from build123d import *

# Parameters (mm, degrees)
F1_DEPTH = 16
F2_R     = 5
F3_DEPTH = 31.200998


with BuildPart() as f1:
    # F0 (on Top) → F1 (new body)
    with BuildSketch(Plane.XY):
        with BuildLine():
            Line((-49.38504, 20.824596), (-48.185041, 20.824596))
            Line((-48.185041, 20.824596), (-48.185041, 36.824596))
            ThreePointArc((-48.185041, 36.824596), (-46.427682, 41.067237), (-42.185041, 42.824596))
            Line((-42.185041, 42.824596), (-18.185041, 42.824596))
            Line((-18.185041, 42.824596), (-18.185041, 44.024594))
            Line((-18.185041, 44.024594), (-42.185041, 44.024594))
            ThreePointArc((-42.185041, 44.024594), (-47.276209, 41.915763), (-49.38504, 36.824596))
            Line((-49.38504, 36.824596), (-49.38504, 20.824596))
        make_face()
    extrude(amount=F1_DEPTH)

    # F2 (on face) → F3 (cut, through all)
    with BuildSketch(Plane(origin=(-49.38504, 0, 0), x_dir=(0, -1, 0), z_dir=(-1, 0, 0))):
        with Locations((-28.824596, 8)):
            Circle(F2_R)
    extrude(amount=-F3_DEPTH, mode=Mode.SUBTRACT)


solid = f1.part
Verification items for the finished model (mm, model axes). A direction names the side the tool comes from. Coordinates: 2 decimals unless noted, no trailing zeros. Loops run counter-clockwise (first coordinate to the right, second up) from the corner with the lowest first, then second, coordinate; pieces in that order, holes last. Notation, with made-up numbers: (48, 2) -> (87, 2) arc R15 ccw to (87, 31) -> close; hole circle Ø4 at (6, 57). An arc over 180 degrees is marked (long way). Answer as a JSON object with one key per item and string values. Group by question number.
Item 1: Mould release check, pull along Z, two halves, no side actions. Record for faces 1 (the flat face through (-43, 43, 16)), 2 (the cylindrical face through (-48.793, 24.055, 9.502)), 3 (the flat face through (-48.185, 25, 4)), 4 (the flat face through (-43, 43, 0)): +Z half, -Z half, draft (parallel to the pull), parting line (faces both ways), or undercut.
Item 2: Sectioned sample at C-C on z = 5.25. Record the boundary of the cut face in (x, y), plus the area to 3 significant figures.
Item 3: Sectioned sample at B-B on y = 31.25. Record the boundary of the cut face in (x, z).
Item 4: Depth check by flat-ended pin: pin 1 (8 mm diameter, centred on y = 30.5, z = 9.5, fed in from +X); pin 2 (1 mm diameter, centred on y = 40.5, z = 12.5, fed in from +X); pin 3 (3 mm diameter, centred on y = 30.5, z = 11, fed in from -X). Enter the tip coordinate at first touch or a pass-through.
Item 5: Scan lines: probe 1 along X at (y, z) = (35.5, 3.25); probe 2 along Y at (x, z) = (-37, 2.5); probe 3 along Y at (x, z) = (-47.5, 5.25). Record each from-to range of solid material in increasing order.
Item 6: Sectioned sample at A-A on z = 8. Record the boundary of the cut face in (x, y).
Item 7: Tool access check on faces 5 (the flat face through (-49.385, 32.5, 4.3)), 6 (the flat face through (-30, 42.825, 8)). Record the directions out of +Z, -Z, +X, -X, +Y, -Y that give a thin tool (end or side, any length) a straight path to the whole face; none if there is none.
Item 8: Sectioned sample at D-D on x = -28. Record the boundary of the cut face in (y, z), plus the area to 3 significant figures.
Evaluation:
{
 "1": {"face 1": "+Z half", "face 2": "undercut", "face 3": "draft", "face 4": "-Z half"},
 "2": {"outline": "(-49.39, 20.82) -> (-48.19, 20.82) -> (-48.19, 24.65) -> (-49.39, 24.65) -> close; (-49.39, 33) -> (-48.19, 33) -> (-48.19, 36.82) arc R6 cw to (-42.19, 42.82) -> (-18.19, 42.82) -> (-18.19, 44.02) -> (-42.19, 44.02) arc R7.2 ccw to (-49.39, 36.82) -> close", "area": "50.4 mm²"},
 "3": {"outline": "(-49.39, 0) -> (-48.19, 0) -> (-48.19, 3.63) -> (-49.39, 3.63) -> close; (-49.39, 12.37) -> (-48.19, 12.37) -> (-48.19, 16) -> (-49.39, 16) -> close"},
 "4": {"pin 1": "stops at x = -48.19", "pin 2": "stops at x = -46.49", "pin 3": "passes through"},
 "5": {"probe 1": "x = -49.39 to -48.19", "probe 2": "y = 42.82 to 44.02", "probe 3": "y = 39.61 to 41.68"},
 "6": {"outline": "(-49.39, 20.82) -> (-48.19, 20.82) -> (-48.19, 23.82) -> (-49.39, 23.82) -> close; (-49.39, 33.82) -> (-48.19, 33.82) -> (-48.19, 36.82) arc R6 cw to (-42.19, 42.82) -> (-18.19, 42.82) -> (-18.19, 44.02) -> (-42.19, 44.02) arc R7.2 ccw to (-49.39, 36.82) -> close"},
 "7": {"face 5": "+Z, -Z, -X, +Y, -Y", "face 6": "+Z, -Z, +X, -Y"},
 "8": {"outline": "(42.82, 0) -> (44.02, 0) -> (44.02, 16) -> (42.82, 16) -> close", "area": "19.2 mm²"}
}
